from build123d import *

# Parameters (mm, degrees)
SKETCH1_R           = 2.8702
BOSS_EXTRUDE1_DEPTH = 6.35
CUT_EXTRUDE1_DEPTH  = 166.459251888


with BuildPart() as part:
    # Sketch1 → Boss-Extrude1 (new body)
    with BuildSketch(Plane.XY):
        Polygon((126.649884677, 0), (113.949884677, 0), (113.949884677, -6.35), (101.249884677, -6.35), (101.249884677, 0), (88.530166142, 0), (88.530166142, -6.35), (88.530166142, -19.145228109), (88.530166142, -51.329150083), (157.167935302, -51.329150083), (157.167935302, -19.145228109), (126.649884677, -19.145228109), (126.649884677, -6.35), align=None)
        with Locations((143.035641266, -34.539684717)):
            Circle(SKETCH1_R, mode=Mode.SUBTRACT)
    extrude(amount=BOSS_EXTRUDE1_DEPTH)

    # Sketch2 → Cut-Extrude1 (cut, through all)
    with BuildSketch(Plane.XY.offset(6.35)):
        with BuildLine():
            Line((143.035641266, -21.547019343), (126.649884677, -19.145228109))
            Line((126.649884677, -19.145228109), (157.167935302, -19.145228109))
            Line((157.167935302, -19.145228109), (157.167935302, -51.329150083))
            Line((157.167935302, -51.329150083), (126.649884677, -51.329150083))
            Line((126.649884677, -51.329150083), (143.035641266, -47.532350091))
            ThreePointArc((143.035641266, -47.532350091), (156.028306641, -34.539684717), (143.035641266, -21.547019343))
        make_face()
    extrude(amount=-CUT_EXTRUDE1_DEPTH, mode=Mode.SUBTRACT)


solid = part.part
Can you work these out from the model? Positions are in its coordinate system, mm. A direction names the side the tool comes from. Coordinates: 2 decimals unless noted, no trailing zeros. Loops run counter-clockwise (first coordinate to the right, second up) from the corner with the lowest first, then second, coordinate; pieces in that order, holes last. Notation, with made-up numbers: M 26,-33.5 L 50,-33.5 A17 ccw 50,-29.5 Z; hole C 13,-30 d4. An arc over 180 degrees is marked long. Return JSON: item names as keys, results as strings. Group by question number.
Item 1: Imagine slicing it at B-B (z = 2.75). Please give me the cut outline in (x, y).
Item 2: If I drill on L1, parallel to X at y = -3, z = 3.75; L2, parallel to X at y = -32.5, z = 1.25; L3, parallel to Y at x = 107, z = 5.5, over which ranges is the centre line in solid material (lowest first)? Write a range as from..to.
Item 3: Thinking about a two-plate mould opening in Y: for faces 4 (the flat face through (134.728, -49.457, 3.219)), 5 (the flat face through (114, -31, 0)), 6 (the cylindrical face through (145.687, -35.639, 3.131)), which applies, released by +Y, released by -Y, zero draft, split by the parting line, or undercut?
Item 4: Imagine slicing it at D-D (x = 106.5). Please give me the cut outline in (y, z), and give its area (3 significant figures).
Item 5: Imagine slicing it at A-A (x = 144). Please give me the cut outline in (y, z), and give its area (3 significant figures).
Item 6: On a 3-axis mill with a long thin cutter (end or side, diameter ignored), from which of +Z, -Z, +X, -X, +Y, -Y can I reach the whole of each face in a straight line? I mean faces 1 (the flat face through (101.25, -3, 3)), 2 (the flat face through (114, -31, 6.35)), 3 (the flat face through (126.65, -10, 3)). Say none if no direction works.
Item 7: Imagine slicing it at C-C (y = -18). Please give me the cut outline in (x, z), and give its area (3 significant figures).
Verdict:
{
 "1": {"outline": "M 88.53,-51.33 L 126.65,-51.33 L 143.04,-47.53 A12.99 ccw 143.04,-21.55 L 126.65,-19.15 L 126.65,0 L 113.95,0 L 113.95,-6.35 L 101.25,-6.35 L 101.25,0 L 88.53,0 Z; hole C 143.04,-34.54 d5.74"},
 "2": {"L1": "x = 88.53..101.25, 113.95..126.65", "L2": "x = 88.53..141.02, 145.05..155.87", "L3": "y = -51.33..-6.35"},
 "3": {"face 4": "released by -Y", "face 5": "zero draft", "face 6": "undercut"},
 "4": {"outline": "M -51.33,0 L -6.35,0 L -6.35,6.35 L -51.33,6.35 Z", "area": "286 mm^2"},
 "5": {"outline": "M -47.5,0 L -37.24,0 L -37.24,6.35 L -47.5,6.35 Z; M -31.84,0 L -21.58,0 L -21.58,6.35 L -31.84,6.35 Z", "area": "130 mm^2"},
 "6": {"face 1": "+Z, -Z, +Y", "face 2": "+Z, +X, -X, +Y, -Y", "face 3": "+Z, -Z, +X, +Y"},
 "7": {"outline": "M 88.53,0 L 126.65,0 L 126.65,6.35 L 88.53,6.35 Z", "area": "242 mm^2"}
}
